from build123d import *

# Parameters (mm, degrees)
F0_W     = 99
F0_H     = 150
F1_DEPTH = 1
F3_DEPTH = 25
F2_R     = 7.5
F2_W     = 32
F2_H     = 22
F4_DEPTH = 25
F5_DEPTH = 25


with BuildPart() as f1:
    # F0 (on Top) → F1 (new body)
    with BuildSketch(Plane.XY):
        Rectangle(F0_W, F0_H)
    extrude(amount=F1_DEPTH)

    # F2 (on face) → F3 (cut)
    with BuildSketch(Plane.XY.offset(1)):
        Polygon((30.116405, 75), (49.5, 47.219642), (49.5, 75), align=None)
        Polygon((-49.5, 47.219642), (-28.743548, 75), (-49.5, 75), align=None)
        Polygon((10.960037, 57.998028), (17.677084, 75), (0, 75), align=None)
        Polygon((23.862131, 62.487412), (30.116405, 75), (17.677084, 75), align=None)
        Polygon((-7.982026, 57.998028), (0, 75), (-16.782477, 75), align=None)
    extrude(amount=-F3_DEPTH, mode=Mode.SUBTRACT)

    # F2 (on face) → F4 (cut)
    with BuildSketch(Plane.XY.offset(1)):
        with Locations((-29.954113, 52.740462)):
            Circle(F2_R)
        with Locations((-33.5, -64)):
            Rectangle(F2_W, F2_H)
        with Locations((33.5, -64)):
            Rectangle(F2_W, F2_H)
        with Locations((28.908281, 52.315958)):
            Circle(F2_R)
    extrude(amount=-F4_DEPTH, mode=Mode.SUBTRACT)

    # F2 (on face) → F5 (cut)
    with BuildSketch(Plane.XY.offset(1)):
        with Locations((33.5, -64)):
            Rectangle(F2_W, F2_H)
        with Locations((-33.5, -64)):
            Rectangle(F2_W, F2_H)
    extrude(amount=-F5_DEPTH, mode=Mode.SUBTRACT)


solid = f1.part
Could you check a few things on this model? Use its own coordinates, in mm. A direction names the side the tool comes from. Coordinates: 2 decimals unless noted, no trailing zeros. Order: outer loops, then holes, each group sorted by start corner. A loop starts at its lowest first (then second) coordinate and runs counter-clockwise, first axis right, second up. Notation, with made-up numbers: (88, 72) - (121, 72) arc R22 cw to (121, 87) - close; hole circle Ø5 at (-25, -1.5). An arc over 180 degrees is marked (long way). Answer in a Markdown table with one row per item. Add a question column.
(1) If we section it at C-C, the plane y = -65: Please give me the cut outline in (x, z), then the cut area to 3 significant figures.
(2) On a 3-axis mill with a long thin cutter (end or side, diameter ignored), from which of +Z, -Z, +X, -X, +Y, -Y can I reach the whole of each face in a straight line? I mean faces 1 (the face through (5.4, 66.62, 0.51)), 2 (the face through (39.673, 61.304, 0.507)). Say none if no direction works.
(3) If we section it at D-D, the plane x = 28: Please give me the cut outline in (y, z), then the cut area to 3 significant figures.
(4) If we mould it in two halves opening along X, with no side actions, what happens to faces 3 (the face through (-23.026, 49.868, 0.507)), 4 (the face through (-12.444, 66.618, 0.507)), 5 (the face through (-39.267, 60.915, 0.507)), 6 (the face through (-1, 1, 0))? For each: released by +X, released by -X, zero draft, split by the parting line, or undercut.
(5) Will these pins go through, and if not, where does the flat tip stop? pin 1 (0.5 mm diameter, centred on y = -59, z = 0.5, fed in from +X); pin 2 (0.5 mm diameter, centred on y = -68.5, z = 0.5, fed in from -X); pin 3 (0.5 mm diameter, centred on x = -32.5, z = 0.5, fed in from -Y).
(6) I need wall thicknesses on L1, parallel to X at y = 64.5, z = 0.5; L2, parallel to Y at x = -27.5, z = 0.5; L3, parallel to X at y = 54, z = 0.7. Which ranges of each line are inside material? Lowest first, please.
(7) If we section it at B-B, the plane z = 0.3: Please give me the cut outline in (x, y), then the cut area to 3 significant figures.
(8) If we section it at A-A, the plane x = -35: Please give me the cut outline in (y, z), then the cut area to 3 significant figures.
Results are:
| question | item | result |
|---|---|---|
| 1 | outline | (-17.5, 0) - (17.5, 0) - (17.5, 1) - (-17.5, 1) - close |
| 1 | area | 35.0 mm2 |
| 2 | face 1 | +Z, -Z, +Y |
| 2 | face 2 | +Z, -Z, +X, +Y |
| 3 | outline | (-53, 0) - (44.87, 0) - (44.87, 1) - (-53, 1) - close; (59.76, 0) - (70.77, 0) - (70.77, 1) - (59.76, 1) - close |
| 3 | area | 109 mm2 |
| 4 | face 3 | undercut |
| 4 | face 4 | undercut |
| 4 | face 5 | released by -X |
| 4 | face 6 | zero draft |
| 5 | pin 1 | stops at x = 17.5 |
| 5 | pin 2 | stops at x = -17.5 |
| 5 | pin 3 | stops at y = -53 |
| 6 | L1 | x = -36.59 to -11.35, -4.93 to 6.77, 13.53 to 22.87, 24.87 to 37.44 |
| 6 | L2 | y = -53 to 45.65, 59.83 to 75 |
| 6 | L3 | x = -44.43 to -37.35, -22.56 to 21.6, 36.22 to 44.77 |
| 7 | outline | (-49.5, -53) - (-17.5, -53) - (-17.5, -75) - (17.5, -75) - (17.5, -53) - (49.5, -53) - (49.5, 47.22) - (30.12, 75) - (23.86, 62.49) - (17.68, 75) - (10.96, 58) - (0, 75) - (-7.98, 58) - (-16.78, 75) - (-28.74, 75) - (-49.5, 47.22) - close; hole circle Ø15 at (-29.95, 52.74); hole circle Ø15 at (28.91, 52.32) |
| 7 | area | 12,200 mm2 |
| 8 | outline | (-53, 0) - (47.19, 0) - (47.19, 1) - (-53, 1) - close; (58.29, 0) - (66.63, 0) - (66.63, 1) - (58.29, 1) - close |
| 8 | area | 109 mm2 |
